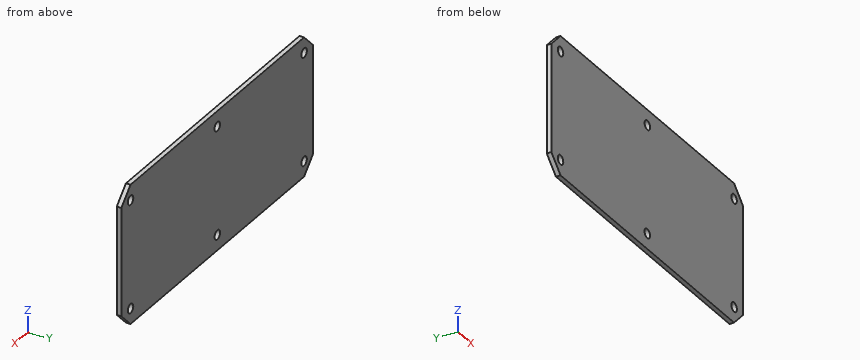
from build123d import *

# Parameters (mm, degrees)
ESQUISSE1_W             = 210
ESQUISSE1_H             = 90
BOSS_EXTRU_1_DEPTH      = 3
ESQUISSE2_R             = 3
ENL_V_MAT_EXTRU_1_DEPTH = 3
CHAMFER1_SIZE           = 10


with BuildPart() as part:
    # Esquisse1 → Boss.-Extru.1 (new body)
    with BuildSketch(Plane(origin=(0, 0, 0), x_dir=(1, 0, 0), z_dir=(0, 1, 0))):
        with Locations((105, 45)):
            Rectangle(ESQUISSE1_W, ESQUISSE1_H)
    extrude(amount=BOSS_EXTRU_1_DEPTH)

    # Esquisse2 → Enlèv. mat.-Extru.1 (cut)
    with BuildSketch(Plane(origin=(0, 3, 0), x_dir=(1, 0, 0), z_dir=(0, 1, 0))):
        with Locations((10, 80)):
            Circle(ESQUISSE2_R)
        with Locations((105, 80)):
            Circle(ESQUISSE2_R)
        with Locations((200, 80)):
            Circle(ESQUISSE2_R)
        with Locations((200, 10)):
            Circle(ESQUISSE2_R)
        with Locations((105, 10)):
            Circle(ESQUISSE2_R)
        with Locations((10, 10)):
            Circle(ESQUISSE2_R)
    extrude(amount=-ENL_V_MAT_EXTRU_1_DEPTH, mode=Mode.SUBTRACT)

    # Chamfer1
    chamfer1_edges = [part.edges().sort_by_distance(p)[0] for p in [
        (210, 1.5, 0),
        (0, 1.5, 0),
        (0, 1.5, -90),
        (210, 1.5, -90),
    ]]
    chamfer(chamfer1_edges, length=CHAMFER1_SIZE)


solid = part.part
The listing builds one solid part. Answer for the finished solid, in the listing's coordinates (mm). Round coordinates to 2 decimals unless told otherwise and drop trailing zeros. Write each loop counter-clockwise with the first axis right and the second up, starting at its lowest first coordinate (ties: lowest second). Pieces come first, ordered by that corner, then holes. Notation, with made-up numbers: (-13, 50.25) - (21, 50.25) arc R11 cw to (21, 55.25) - close; hole circle Ø7 at (57.25, 29). An arc over 180 degrees is marked (long way). Use a Markdown table: item, result. Add a question column.
1. Consider line 1 (X direction, y = 2.2, z = -10); line 2 (Z direction, x = 105, y = 1.55); line 3 (X direction, y = 1, z = -79). Determine where each line is inside the solid, lowest interval first.
2. The part is cut by section B-B (y = 2.1). Write down the section's boundary in (x, z).
3. The part is cut by section A-A (x = 105). Write down the section's boundary in (y, z).
Reported:
| question | item | result |
|---|---|---|
| 1 | line 1 | 0 to 7, 13 to 102, 108 to 197, 203 to 210 |
| 1 | line 2 | -90 to -83, -77 to -13, -7 to 0 |
| 1 | line 3 | 0 to 7.17, 12.83 to 102.17, 107.83 to 197.17, 202.83 to 210 |
| 2 | outline | (0, -80) - (10, -90) - (200, -90) - (210, -80) - (210, -10) - (200, 0) - (10, 0) - (0, -10) - close; hole circle Ø6 at (10, -80); hole circle Ø6 at (10, -10); hole circle Ø6 at (105, -80); hole circle Ø6 at (105, -10); hole circle Ø6 at (200, -80); hole circle Ø6 at (200, -10) |
| 3 | outline | (0, -90) - (3, -90) - (3, -83) - (0, -83) - close; (0, -77) - (3, -77) - (3, -13) - (0, -13) - close; (0, -7) - (3, -7) - (3, 0) - (0, 0) - close |
